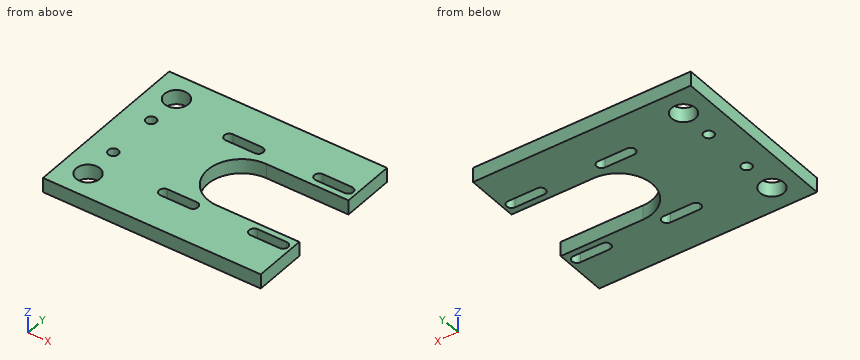
```python
from build123d import *

# Parameters (mm, degrees)
SKETCH1_W           = 5
SKETCH1_H           = 60
BOSS_EXTRUDE1_DEPTH = 5
SKETCH2_W           = 5
SKETCH2_H           = 60
BOSS_EXTRUDE2_DEPTH = 50
CUT_EXTRUDE4_DEPTH  = 6
CUT_EXTRUDE5_DEPTH  = 6
SKETCH7_W           = 5
SKETCH7_H           = 60
BOSS_EXTRUDE3_DEPTH = 20
SKETCH8_R           = 4.1
SKETCH8_R_2         = 1.75
CUT_EXTRUDE6_DEPTH  = 6


with BuildPart() as part:
    # Sketch1 → Boss-Extrude1 (new body)
    with BuildSketch(Plane(origin=(0, 0, 0), x_dir=(0, 0, -1), z_dir=(1, 0, 0))):
        with Locations((-36.107304337, -1.744616853)):
            Rectangle(SKETCH1_W, SKETCH1_H)
    extrude(amount=BOSS_EXTRUDE1_DEPTH)

    # Sketch2 → Boss-Extrude2 (add)
    with BuildSketch(Plane(origin=(5, 0, 0), x_dir=(0, 0, -1), z_dir=(1, 0, 0))):
        with Locations((-36.107304337, -1.744616853)):
            Rectangle(SKETCH2_W, SKETCH2_H)
    extrude(amount=BOSS_EXTRUDE2_DEPTH)

    # Sketch5 → Cut-Extrude4 (cut, through all)
    with BuildSketch(Plane(origin=(0, 0, 33.607304337), x_dir=(-1, 0, 0), z_dir=(0, 0, -1))):
        with BuildLine():
            Line((-26.7, -13.444616853), (-56.7, -13.444616853))
            ThreePointArc((-56.7, -13.444616853), (-68.4, -1.744616853), (-56.7, 9.955383147))
            Line((-56.7, 9.955383147), (-26.7, 9.955383147))
            ThreePointArc((-26.7, 9.955383147), (-15, -1.744616853), (-26.7, -13.444616853))
        make_face()
    extrude(amount=-CUT_EXTRUDE4_DEPTH, mode=Mode.SUBTRACT)

    # Sketch6 → Cut-Extrude5 (cut, through all)
    with BuildSketch(Plane(origin=(0, 0, 33.607304337), x_dir=(-1, 0, 0), z_dir=(0, 0, -1))):
        with BuildLine():
            Line((-42.2, 12.055383147), (-52.2, 12.055383147))
            ThreePointArc((-52.2, 12.055383147), (-53.9, 13.755383147), (-52.2, 15.455383147))
            Line((-52.2, 15.455383147), (-42.2, 15.455383147))
            ThreePointArc((-42.2, 15.455383147), (-40.5, 13.755383147), (-42.2, 12.055383147))
        make_face()
        with BuildLine():
            Line((-42.2, -18.944616853), (-52.2, -18.944616853))
            ThreePointArc((-52.2, -18.944616853), (-53.9, -17.244616853), (-52.2, -15.544616853))
            Line((-52.2, -15.544616853), (-42.2, -15.544616853))
            ThreePointArc((-42.2, -15.544616853), (-40.5, -17.244616853), (-42.2, -18.944616853))
        make_face()
        with BuildLine():
            Line((-11.2, -18.944616853), (-21.2, -18.944616853))
            ThreePointArc((-21.2, -18.944616853), (-22.9, -17.244616853), (-21.2, -15.544616853))
            Line((-21.2, -15.544616853), (-11.2, -15.544616853))
            ThreePointArc((-11.2, -15.544616853), (-9.5, -17.244616853), (-11.2, -18.944616853))
        make_face()
        with BuildLine():
            Line((-11.2, 12.055383147), (-21.2, 12.055383147))
            ThreePointArc((-21.2, 12.055383147), (-22.9, 13.755383147), (-21.2, 15.455383147))
            Line((-21.2, 15.455383147), (-11.2, 15.455383147))
            ThreePointArc((-11.2, 15.455383147), (-9.5, 13.755383147), (-11.2, 12.055383147))
        make_face()
    extrude(amount=-CUT_EXTRUDE5_DEPTH, mode=Mode.SUBTRACT)

    # Sketch7 → Boss-Extrude3 (add)
    with BuildSketch(Plane.ZY):
        with Locations((36.107304337, -1.744616853)):
            Rectangle(SKETCH7_W, SKETCH7_H)
    extrude(amount=BOSS_EXTRUDE3_DEPTH)

    # Sketch8 → Cut-Extrude6 (cut, through all)
    with BuildSketch(Plane(origin=(0, 0, 33.607304337), x_dir=(-1, 0, 0), z_dir=(0, 0, -1))):
        with Locations((11, 19.255383147)):
            Circle(SKETCH8_R)
        with Locations((11, -22.744616853)):
            Circle(SKETCH8_R)
        with Locations((11, -10.744616853)):
            Circle(SKETCH8_R_2)
        with Locations((11, 7.255383147)):
            Circle(SKETCH8_R_2)
    extrude(amount=-CUT_EXTRUDE6_DEPTH, mode=Mode.SUBTRACT)


solid = part.part
```
CAD build for the part. Positions are in the model's coordinates, mm. Round coordinates to 2 decimals unless told otherwise and drop trailing zeros. Loops run counter-clockwise (first coordinate to the right, second up) from the corner with the lowest first, then second, coordinate; pieces in that order, holes last. Notation, with made-up numbers: M 3,51 L 49,51 A35 ccw 49,89 Z; hole C -27,50 d9. An arc over 180 degrees is marked long. Return JSON: item names as keys, results as strings. Group by question number.
(1) Saw through at C-C, the plane z = 35.55. Give the number of separate pieces and of enclosed holes in the cut face, and give its area (3 significant figures).
(2) Saw through at A-A, the plane x = 50. List the corners of the cut face in (y, z), and give its area (3 significant figures).
(3) Saw through at B-B, the plane x = -11. List the corners of the cut face in (y, z), and give its area (3 significant figures).
(4) Wall check: probe 1 along Y at (x, z) = (-11, 35.6); probe 2 along Y at (x, z) = (48, 36.8); probe 3 along Y at (x, z) = (-10, 37.2). Give the ranges that are in metal, low to high. Write a range as [from, to].
(5) Saw through at D-D, the plane x = 25. List the corners of the cut face in (y, z), and give its area (3 significant figures).
Answer list:
{
 "1": {"separate pieces": "1", "enclosed holes": "8", "area": "3,330 mm2"},
 "2": {"outline": "M -31.74,33.61 L -18.94,33.61 L -18.94,38.61 L -31.74,38.61 Z; M -15.54,33.61 L -13.44,33.61 L -13.44,38.61 L -15.54,38.61 Z; M 9.96,33.61 L 12.06,33.61 L 12.06,38.61 L 9.96,38.61 Z; M 15.46,33.61 L 28.26,33.61 L 28.26,38.61 L 15.46,38.61 Z", "area": "149 mm2"},
 "3": {"outline": "M -31.74,33.61 L -26.84,33.61 L -26.84,38.61 L -31.74,38.61 Z; M -18.64,33.61 L -12.49,33.61 L -12.49,38.61 L -18.64,38.61 Z; M -8.99,33.61 L 5.51,33.61 L 5.51,38.61 L -8.99,38.61 Z; M 9.01,33.61 L 15.16,33.61 L 15.16,38.61 L 9.01,38.61 Z; M 23.36,33.61 L 28.26,33.61 L 28.26,38.61 L 23.36,38.61 Z", "area": "183 mm2"},
 "4": {"probe 1": "[-31.74, -26.84], [-18.64, -12.49], [-8.99, 5.51], [9.01, 15.16], [23.36, 28.26]", "probe 2": "[-31.74, -18.94], [-15.54, -13.44], [9.96, 12.06], [15.46, 28.26]", "probe 3": "[-31.74, -26.72], [-18.77, -12.18], [-9.31, 5.82], [8.69, 15.28], [23.23, 28.26]"},
 "5": {"outline": "M -31.74,33.61 L -13.32,33.61 L -13.32,38.61 L -31.74,38.61 Z; M 9.83,33.61 L 28.26,33.61 L 28.26,38.61 L 9.83,38.61 Z", "area": "184 mm2"}
}
